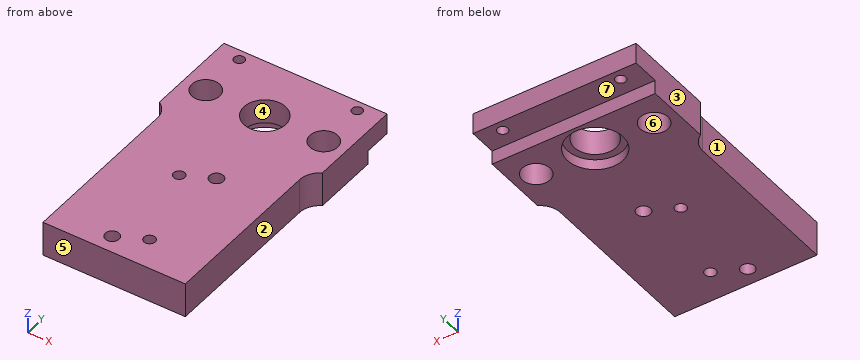
Autodesk Inventor part; units mm, degrees
ref_plane "YZ Plane" through (0, 0, 0) normal (1, 0, 0) x (0, 1, 0)
ref_plane "XZ Plane" through (0, 0, 0) normal (0, 1, 0) x (-1, 0, 0)
ref_plane "XY Plane" through (0, 0, 0) normal (0, 0, 1) x (1, 0, 0)
sketch "Sketch1" plane through (0, 0, 0) normal (0, 0, 1) x (1, 0, 0)
  line L0 (0, 40) -> (0, -40)
  line L1 (0, 40) -> (23.5, 40)
  line L2 (23.5, 40) -> (23.5, 13)
  arc A0 (23.5, 13) -> (20.5, 7.8038) centre (26.5, 7.8038) ccw
  line L3 (20.5, 7.8038) -> (20.5, -40)
  line L4 (20.5, -40) -> (0, -40)
  line L5 (0, 40) -> (-23.5, 40)
  line L6 (-23.5, 40) -> (-23.5, 13)
  arc A1 (-20.5, 7.8038) -> (-23.5, 13) centre (-26.5, 7.8038) ccw
  line L7 (-20.5, 7.8038) -> (-20.5, -40)
  line L8 (-20.5, -40) -> (0, -40)
  point P0 (0, 0)
  point P1 (0, 0)
  point P2 (10.25, -40)
  dimension "d0" = 47
  dimension "d1" = 80
  dimension "d2" = 27
  dimension "d3" = 41
  dimension "d4" = 6
extrude "Extrusion1" add sketch "Sketch1" along normal mid plane 10
sketch "Sketch2" plane through (23.5, 13, 5) normal (1, 0, 0) x (0, 0, -1)
  line L0 (10, 27) -> (0, 27)
  line L1 (6, 27) -> (6, 19)
  line L2 (6, 19) -> (10, 19)
  line L3 (10, 27) -> (10, 0)
  point P0 (5, -13)
  dimension "d7" = 8
  dimension "d8" = 4
extrude "Extrusion2" cut sketch "Sketch2" against normal through all
sketch "Sketch3" plane through (0, 0, -5) normal (0, 0, -1) x (-1, 0, 0)
  line L0 (-23.5, 40) -> (23.5, 40)
  line L1 (0, 40) -> (0, -40)
  line L2 (-20.5, -40) -> (20.5, -40)
  line L3 (-20.5, 7.8038) -> (-20.5, -40)
  point P0 (0, 0)
  point P1 (-17, 23)
  point P2 (0, 23)
  point P3 (17, 23)
  point P4 (-4, -3)
  point P5 (4, -7)
  point P6 (-4, -31)
  point P7 (4, -35)
  dimension "d11" = 17
  dimension "d12" = 34
  dimension "d13" = 5
  dimension "d14" = 32
  dimension "d15" = 4
  dimension "d16" = 24
  dimension "d17" = 16.5
  dimension "d18" = 24.5
hole "Hole1" at (-4, -35, -5) at (4, -3, -5) direction (0, 0, 1) diameter 4 end through all
hole "Hole2" at (4, -31, -5) at (-4, -7, -5) direction (0, 0, 1) diameter 3.242 end through all
hole "Hole3" at (17, 23, -5) at (-17, 23, -5) direction (0, 0, 1) diameter 8 end through all
hole "Hole4" at (0, 23, -5) direction (0, 0, 1) diameter 12 end through all counterbore diameter 16 counterbore depth 3
sketch "Sketch5" plane through (23.5, 32, -1) normal (0, 0, -1) x (-1, 0, 0)
  line L0 (0, 8) -> (47, 8)
  line L1 (23.5, 8) -> (23.5, 5)
  line L2 (23.5, 5) -> (40.5, 5)
  line L3 (40.5, 5) -> (6.5, 5)
  circle A0 centre (6.5, 5) radius 1.5
  circle A1 centre (40.5, 5) radius 1.5
  point P0 (23.5, -32)
  dimension "d58" = 3
  dimension "d59" = 17
  dimension "d60" = 34
  dimension "d61" = 3
  dimension "d62" = 3
extrude "Extrusion4" cut sketch "Sketch5" against normal blind 10
properties part number "Lap2" material "Steel, Carbon"
Could you check a few things on this model? Use its own coordinates, in mm. Face numbers are marked on the shaded views. A direction names the side the tool comes from. Give positions to 0.01 mm unless a question says otherwise; leave off trailing zeros. Write each loop counter-clockwise with the first axis right and the second up, starting at its lowest first coordinate (ties: lowest second). Pieces come first, ordered by that corner, then holes. Notation, with made-up numbers: (-17, 36.5) - (12, 36.5) arc R27 cw to (12, 69.5) - close; hole circle Ø5 at (81, 5.5). An arc over 180 degrees is marked (long way). One line per item, written item: value. Start each with the question number.
Item 1: Imagine slicing it at C-C, the plane y = -3. List the corners of the cut face in (x, z) for me, and give its area (3 significant figures).
Item 2: Please list where these lines run through material, in increasing order: line 1 (Y direction, x = 17, z = 3); line 2 (X direction, y = 23, z = 2.25); line 3 (X direction, y = -35, z = -0.5). Write a range as from..to.
Item 3: Imagine slicing it at D-D, the plane z = 2. Give the number of separate pieces and of enclosed holes in the cut face, and give its area (3 significant figures).
Item 4: Which directions (+Z, -Z, +X, -X, +Y, -Y) give clear straight access to the entire face, cutting with the end or side of a thin tool? Please do the marked faces 1, 2 and 3.
Item 5: Imagine slicing it at A-A, the plane x = 17. List the corners of the cut face in (y, z) for me.
Item 6: If we mould it in two halves opening along Y, with no side actions, what happens to the marked faces 4, 5, 6 and 7? For each: +Y half, -Y half, draft (parallel to the pull), parting line (faces both ways), or undercut.
Item 7: I'm going to push flat-ended pins straight in: pin 1 (6 mm diameter, centred on y = -28, z = -0.5, fed in from +X); pin 2 (2.5 mm diameter, centred on x = 4, y = -31, fed in from -Z); pin 3 (1 mm diameter, centred on y = -23, z = 0, fed in from -X); pin 4 (3.5 mm diameter, centred on x = 17, y = 37, fed in from -Z). Where does each tip first touch, or does it pass through?
Item 8: Imagine slicing it at B-B, the plane z = -4. List the corners of the cut face in (x, y) for me.
Geometry says:
1. outline: (-20.5, -5) - (2, -5) - (2, 5) - (-20.5, 5) - close; (6, -5) - (20.5, -5) - (20.5, 5) - (6, 5) - close
1. area: 370 mm^2
2. line 1: -40..19, 27..35.5, 38.5..40
2. line 2: -23.5..-21, -13..-6, 6..13, 21..23.5
2. line 3: -20.5..-6, -2..20.5
3. separate pieces: 1
3. enclosed holes: 9
3. area: 3,180 mm^2
4. face 1: +Z, -Z, -X, -Y
4. face 2: +Z, -Z, +X, -Y
4. face 3: +Z, -Z, -X, +Y, -Y
5. outline: (-40, -5) - (19, -5) - (19, 5) - (-40, 5) - close; (27, -5) - (32, -5) - (32, -1) - (35.5, -1) - (35.5, 5) - (27, 5) - close; (38.5, -1) - (40, -1) - (40, 5) - (38.5, 5) - close
6. face 4: undercut
6. face 5: -Y half
6. face 6: undercut
6. face 7: draft
7. pin 1: x = 20.5
7. pin 2: through
7. pin 3: x = -20.5
7. pin 4: z = -1
8. outline: (-23.5, 13) arc R6 cw to (-20.5, 7.8) - (-20.5, -40) - (20.5, -40) - (20.5, 7.8) arc R6 cw to (23.5, 13) - (23.5, 32) - (-23.5, 32) - close; hole circle Ø8 at (-17, 23); hole circle Ø16 at (0, 23); hole circle Ø4 at (-4, -35); hole circle Ø3.24 at (-4, -7); hole circle Ø4 at (4, -3); hole circle Ø3.24 at (4, -31); hole circle Ø8 at (17, 23)
